from build123d import *

# Parameters (mm, degrees)
CROQUIS1_W              = 70
CROQUIS1_H              = 34
CROQUIS1_R              = 11.2
CROQUIS1_R_2            = 4.1
SALIENTE_EXTRUIR1_DEPTH = 9
CROQUIS2_W              = 70
CROQUIS2_H              = 34
CROQUIS2_R              = 5.5
SALIENTE_EXTRUIR2_DEPTH = 8
CUT_EXTRUDE1_REACH      = 92.756
CUT_EXTRUDE1_END_RADIUS = 4.1
SKETCH1_R               = 1.5
CUT_EXTRUDE2_REACH      = 92.756
CUT_EXTRUDE2_END_RADIUS = 4.1
SKETCH2_R               = 1.5
FILLET1_R               = 4


with BuildPart() as part:
    # Croquis1 → Saliente-Extruir1 (new body)
    with BuildSketch(Plane.XY):
        with Locations((229.019677403, 38.205269585)):
            Rectangle(CROQUIS1_W, CROQUIS1_H)
        with Locations((229.019677403, 38.205269585)):
            Circle(CROQUIS1_R, mode=Mode.SUBTRACT)
        with Locations((201.319677403, 38.205269585)):
            Circle(CROQUIS1_R_2, mode=Mode.SUBTRACT)
        with Locations(Location((256.719677403, 38.205269585, 0), (0, 0, 180))):
            Circle(CROQUIS1_R_2, mode=Mode.SUBTRACT)
    extrude(amount=SALIENTE_EXTRUIR1_DEPTH)

    # Croquis2 → Saliente-Extruir2 (add)
    with BuildSketch(Plane.XY.offset(9)):
        with Locations((229.019677403, 38.205269585)):
            Rectangle(CROQUIS2_W, CROQUIS2_H)
        with Locations((229.019677403, 38.205269585)):
            Circle(CROQUIS2_R, mode=Mode.SUBTRACT)
    extrude(amount=SALIENTE_EXTRUIR2_DEPTH)

    # Cut-Extrude1: up to this cylinder (the profile starts outside it)
    cut_extrude1_end = Plane(origin=(201.319677403, 38.205269585, 5), z_dir=(0, 0, -1)) * Cylinder(CUT_EXTRUDE1_END_RADIUS, 194.712, mode=Mode.PRIVATE)
    # Sketch1 → Cut-Extrude1 (cut, up to the surface)
    with BuildSketch(Plane.ZY.offset(-194.019677403), mode=Mode.PRIVATE) as cut_extrude1_sk1:
        with Locations((5, 37.981969781)):
            Circle(SKETCH1_R)
    cut_extrude1_tool1 = extrude(cut_extrude1_sk1.sketch, amount=-CUT_EXTRUDE1_REACH, mode=Mode.PRIVATE) - cut_extrude1_end
    add(cut_extrude1_tool1.solids().sort_by_distance((194.019677, 37.98197, 5))[0], mode=Mode.SUBTRACT)

    # Cut-Extrude2: up to this cylinder (the profile starts outside it)
    cut_extrude2_end = Plane(origin=(256.719677403, 38.205269585, 5), z_dir=(0, 0, -1)) * Cylinder(CUT_EXTRUDE2_END_RADIUS, 194.712, mode=Mode.PRIVATE)
    # Sketch2 → Cut-Extrude2 (cut, up to the surface)
    with BuildSketch(Plane(origin=(264.019677403, 0, 0), x_dir=(0, 0, -1), z_dir=(1, 0, 0)), mode=Mode.PRIVATE) as cut_extrude2_sk1:
        with Locations((-5, 38.205269585)):
            Circle(SKETCH2_R)
    cut_extrude2_tool1 = extrude(cut_extrude2_sk1.sketch, amount=-CUT_EXTRUDE2_REACH, mode=Mode.PRIVATE) - cut_extrude2_end
    add(cut_extrude2_tool1.solids().sort_by_distance((264.019677, 38.20527, 5))[0], mode=Mode.SUBTRACT)

    # Fillet1
    fillet1_edges = [part.edges().sort_by_distance(p)[0] for p in [
        (194.019677403, 55.205269585, 8.5),
        (264.019677403, 55.205269585, 8.5),
        (264.019677403, 21.205269585, 8.5),
        (194.019677403, 21.205269585, 8.5),
    ]]
    fillet(fillet1_edges, radius=FILLET1_R)


solid = part.part
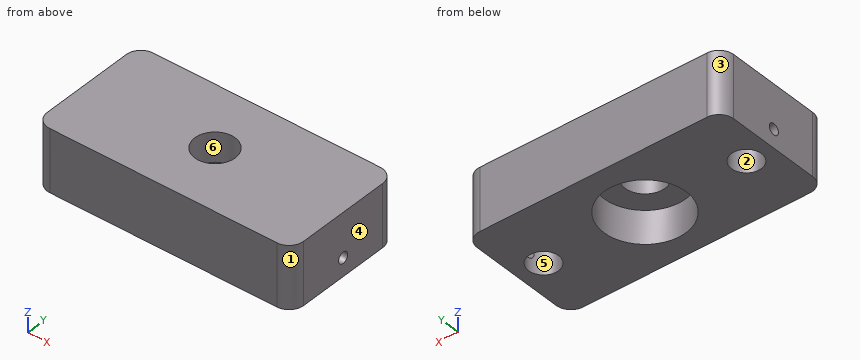
Source: CAD feature listing. Evaluate the final solid. Frame: model axes, mm. Face numbers are marked on the shaded views. A direction names the side the tool comes from. Give positions to 0.01 mm unless a question says otherwise; leave off trailing zeros. Loops run counter-clockwise (first coordinate to the right, second up) from the corner with the lowest first, then second, coordinate; pieces in that order, holes last. Notation, with made-up numbers: (35.25, 65.5) -> (62.25, 65.5) arc R21 cw to (62.25, 91.5) -> close; hole circle Ø11 at (55, 46). An arc over 180 degrees is marked (long way). Use a Markdown table: item, result. Add a question column.
1) Section query C-C, the plane z = 1.5. Return the cut outline in (x, y), then the cut area to 3 significant figures.
2) Section query A-A, the plane x = 231. Return the cut outline in (y, z), then the cut area to 3 significant figures.
3) Line query: line 1 along X through (y, z) = (41.5, 4.5); line 2 along X through (y, z) = (41, 6.5); line 3 along Y through (x, z) = (261.9, 5). Output: solid intervals per line, ascending. Write a range as [from, to].
4) Section query B-B, the plane z = 5. Return the cut outline in (x, y), then the cut area to 3 significant figures.
5) Section query D-D, the plane y = 48.5. Return the cut outline in (x, z).
6) Pull-direction query (Y, two-part tool) for the marked faces 1, 2, 3 and 4; classes: +Y half, -Y half, draft (parallel to the pull), parting line (faces both ways), or undercut.
7) First-contact query: pin 1 (7.5 mm diameter, centred on x = 256.72, y = 38.21, fed in from -Z). Flat tip, straight axial feed; report the tip coordinate or a pass-through.
8) Reachability of the marked faces 5 and 6 from +Z, -Z, +X, -X, +Y, -Y: full face, straight path, thin tool, end or side. Return the list, or none.
Numbers:
| question | item | result |
|---|---|---|
| 1 | outline | (194.02, 25.21) arc R4 ccw to (198.02, 21.21) -> (260.02, 21.21) arc R4 ccw to (264.02, 25.21) -> (264.02, 51.21) arc R4 ccw to (260.02, 55.21) -> (198.02, 55.21) arc R4 ccw to (194.02, 51.21) -> close; hole circle Ø8.2 at (201.32, 38.21); hole circle Ø22.4 at (229.02, 38.21); hole circle Ø8.2 at (256.72, 38.21) |
| 1 | area | 1,870 mm2 |
| 2 | outline | (21.21, 0) -> (27.18, 0) -> (27.18, 9) -> (33.07, 9) -> (33.07, 17) -> (21.21, 17) -> close; (43.34, 9) -> (49.23, 9) -> (49.23, 0) -> (55.21, 0) -> (55.21, 17) -> (43.34, 17) -> close |
| 2 | area | 297 mm2 |
| 3 | line 1 | x = [194.02, 198.88], [203.76, 218.32], [239.72, 254.28], [259.16, 264.02] |
| 3 | line 2 | x = [194.02, 198.32], [204.32, 218.17], [239.87, 253.72], [259.72, 264.02] |
| 3 | line 3 | y = [21.67, 36.71], [39.71, 54.74] |
| 4 | outline | (194.02, 25.21) arc R4 ccw to (198.02, 21.21) -> (260.02, 21.21) arc R4 ccw to (264.02, 25.21) -> (264.02, 36.71) -> (260.54, 36.71) arc R4.1 cw (long way) to (260.54, 39.71) -> (264.02, 39.71) -> (264.02, 51.21) arc R4 ccw to (260.02, 55.21) -> (198.02, 55.21) arc R4 ccw to (194.02, 51.21) -> (194.02, 39.48) -> (197.42, 39.48) arc R4.1 cw (long way) to (197.6, 36.48) -> (194.02, 36.48) -> close; hole circle Ø22.4 at (229.02, 38.21) |
| 4 | area | 1,850 mm2 |
| 5 | outline | (194.02, 0) -> (224.61, 0) -> (224.61, 9) -> (233.43, 9) -> (233.43, 0) -> (264.02, 0) -> (264.02, 17) -> (194.02, 17) -> close |
| 6 | face 1 | -Y half |
| 6 | face 2 | undercut |
| 6 | face 3 | +Y half |
| 6 | face 4 | draft |
| 7 | pin 1 | stops at z = 9 |
| 8 | face 5 | -Z |
| 8 | face 6 | +Z, -Z |
